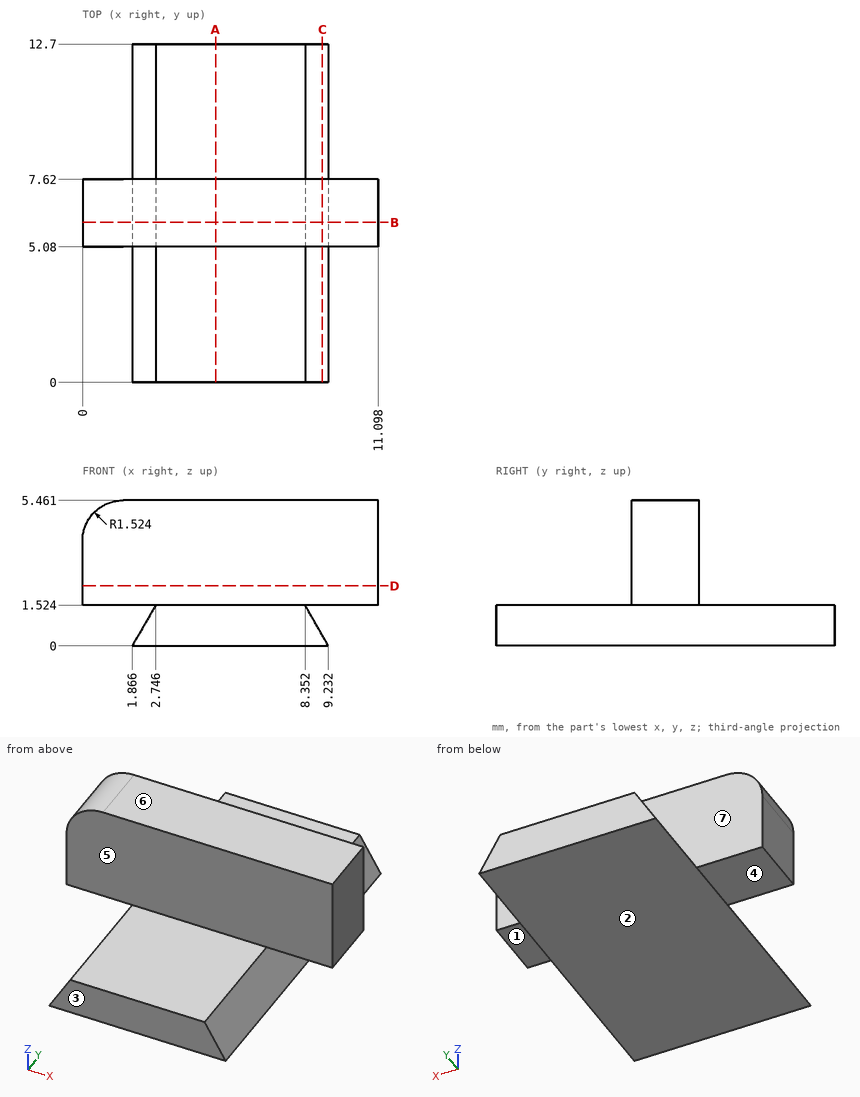
Here's the drawing with two shaded views (mm, measured from the low corner). I have some questions. A direction names the side the tool comes from. Coordinates: 2 decimals unless noted, no trailing zeros. Loops run counter-clockwise (first coordinate to the right, second up) from the corner with the lowest first, then second, coordinate; pieces in that order, holes last.
Item 1: Suppose I cut it at D-D (z = 2.25). Please give me the cut outline in (x, y).
Answers below:
outline: (0, 5.08) - (11.1, 5.08) - (11.1, 7.62) - (0, 7.62) - close
Item 2: Suppose I cut it at C-C (x = 9). Please give me the cut outline in (y, z).
Answers below:
outline: (0, 0) - (12.7, 0) - (12.7, 0.4) - (0, 0.4) - close; (5.08, 1.52) - (7.62, 1.52) - (7.62, 5.46) - (5.08, 5.46) - close
Item 3: Which directions (+Z, -Z, +X, -X, +Y, -Y) give clear straight access to the entire face, cutting with the end or side of a thin tool? Please do the marked faces 5, 6 and 7.
Answers below:
face 5: +Z, +X, -X, -Y
face 6: +Z, +X, -X, +Y, -Y
face 7: +Z, +X, -X, +Y
Item 4: If we mould it in two halves opening along Z, with no side actions, what happens to the marked faces 1, 2, 3 and 4? For each: released by +Z, released by -Z, zero draft, split by the parting line, or undercut.
Answers below:
face 1: undercut
face 2: released by -Z
face 3: zero draft
face 4: undercut
Item 5: I'm going to push flat-ended pins straight in: pin 1 (5.5 mm diameter, centred on x = 4.5, y = 1.5, fed in from +Z); pin 2 (2 mm diameter, centred on x = 10.5, y = 6.5, fed in from -Z); pin 3 (1.2 mm diameter, centred on x = 6.5, z = 3.5, fed in from +Y); pin 4 (1.5 mm diameter, centred on y = 8.5, z = 3.5, fed in from -X). Where does each tip first touch, or does it pass through?
Answers below:
pin 1: stops at z = 1.52
pin 2: stops at z = 1.52
pin 3: stops at y = 7.62
pin 4: passes through
Item 6: Please list where these lines run through material, in increasing order: L1, parallel to Y at x = 8.25, z = 3; L2, parallel to Z at x = 2.25, y = 5.5 (1 decimal); L3, parallel to Z at x = 8, y = 5.
Answers below:
L1: y = 5.08 to 7.62
L2: z = 0 to 0.7, 1.5 to 5.5
L3: z = 0 to 1.52
Item 7: Suppose I cut it at B-B (y = 6). Please give me the cut outline in (x, z).
Answers below:
outline: (0, 1.52) - (2.75, 1.52) - (1.87, 0) - (9.23, 0) - (8.35, 1.52) - (11.1, 1.52) - (11.1, 5.46) - (1.52, 5.46) arc R1.52 ccw to (0, 3.94) - close
Item 8: Suppose I cut it at A-A (x = 5). Please give me the cut outline in (y, z).
Answers below:
outline: (0, 0) - (12.7, 0) - (12.7, 1.52) - (7.62, 1.52) - (7.62, 5.46) - (5.08, 5.46) - (5.08, 1.52) - (0, 1.52) - close
